Design review of the part built by this model. Coordinates are the model's own, in mm. A direction names the side the tool comes from. Coordinates: 2 decimals unless noted, no trailing zeros. Loops run counter-clockwise (first coordinate to the right, second up) from the corner with the lowest first, then second, coordinate; pieces in that order, holes last. Notation, with made-up numbers: (20, 22) - (37, 22) arc R21 cw to (37, 56) - close; hole circle Ø7 at (64, 64.25). An arc over 180 degrees is marked (long way). Answer in a Markdown table with one row per item. Add a question column.
(1) The part is to be moulded in two halves that separate along Z. For faces 3 (the face through (-19.524, 2.021, -4.336)), 4 (the face through (0, 5.6, 0)), 5 (the face through (-10.8, 2.8, -5.7)), say which applies: released by +Z, released by -Z, zero draft, split by the parting line, or undercut.
(2) We need section B-B, the plane y = 2.5. Write out the cut boundary in (x, z).
(3) We need section A-A, the plane x = 0. Write out the cut boundary in (y, z), plus the area to 3 significant figures.
(4) To check wall thickness, follow L1, parallel to X at y = 1.25, z = -6; L2, parallel to Z at x = 8, y = 4; L3, parallel to Z at x = 9.5, y = 1.8. State the ranges of each line that lie inside material, in increasing order. Write a range as [from, to].
(5) We need section D-D, the plane z = -9. Write out the cut boundary in (x, y), plus the area to 3 significant figures.
(6) Clearance check with flat-ended pins moving along their axes: pin 1 (3.5 mm diameter, centred on x = 0, z = 10, fed in from -Y); pin 2 (2 mm diameter, centred on x = -5.5, y = 2.5, fed in from -Z); pin 3 (3 mm diameter, centred on y = 2, z = -10.5, fed in from +X); pin 4 (1.5 mm diameter, centred on x = 3, y = 4.5, fed in from +Z). State where each tip first meets the part, or that it passes through.
(7) For faces 1 (the face through (-15.62, 4.84, -3.47)), 2 (the face through (0, 0, 0)), list the 3-axis set-ups (+Z, -Z, +X, -X, +Y, -Y) from which the entire face can be reached by the end or side of a thin tool; tool diameter is ignored.
(8) We need section C-C, the plane z = 0. Write out the cut boundary in (x, y).
from build123d import *

# Parameters (mm, degrees)
SKIZZE1_R                       = 20
AUFSATZ_LINEAR_AUSTRAGEN1_DEPTH = 5.6
SCHNITT_LINEAR_START            = -1.5
SKIZZE2_R                       = 20
SKIZZE2_R_2                     = 16
SCHNITT_LINEAR_AUSTRAGEN1_DEPTH = 1.5
DURCHGANGSLOCH_F_R_M41_D        = 4.5


with BuildPart() as part:
    # Skizze1 → Aufsatz-Linear austragen1 (new body)
    with BuildSketch(Plane(origin=(0, 0, 0), x_dir=(1, 0, 0), z_dir=(0, 1, 0))):
        with Locations(Location((0, 0, 0), (0, 0, 270))):
            Circle(SKIZZE1_R)
    extrude(amount=AUFSATZ_LINEAR_AUSTRAGEN1_DEPTH)

    # Skizze2 → Schnitt-Linear austragen1 (cut)
    with BuildSketch(Plane(origin=(0, 5.6, 0), x_dir=(1, 0, 0), z_dir=(0, 1, 0)).offset(SCHNITT_LINEAR_START)):
        with Locations(Location((0, 0, 0), (0, 0, 270))):
            Circle(SKIZZE2_R)
        with Locations(Location((0, 0, 0), (0, 0, 270))):
            Circle(SKIZZE2_R_2, mode=Mode.SUBTRACT)
    extrude(amount=SCHNITT_LINEAR_AUSTRAGEN1_DEPTH, mode=Mode.SUBTRACT)

    # Durchgangsloch für M41 (through all)
    with Locations(Plane(origin=(0, 5.6, 0), x_dir=(1, 0, 0), z_dir=(0, 1, 0))):
        with Locations((0, 10), (8.660254038, 5), (8.660254038, -5), (0, -10), (-8.660254038, -5), (-8.660254038, 5)):
            Hole(DURCHGANGSLOCH_F_R_M41_D / 2)


solid = part.part
Responses:
| question | item | result |
|---|---|---|
| 1 | face 3 | split by the parting line |
| 1 | face 4 | zero draft |
| 1 | face 5 | undercut |
| 2 | outline | circle Ø40 at (0, 0); hole circle Ø4.5 at (-8.66, -5); hole circle Ø4.5 at (-8.66, 5); hole circle Ø4.5 at (0, -10); hole circle Ø4.5 at (0, 10); hole circle Ø4.5 at (8.66, -5); hole circle Ø4.5 at (8.66, 5) |
| 3 | outline | (0, -20) - (4.1, -20) - (4.1, -16) - (5.6, -16) - (5.6, -12.25) - (0, -12.25) - close; (0, -7.75) - (5.6, -7.75) - (5.6, 7.75) - (0, 7.75) - close; (0, 12.25) - (5.6, 12.25) - (5.6, 16) - (4.1, 16) - (4.1, 20) - (0, 20) - close |
| 3 | area | 162 mm2 |
| 4 | L1 | x = [-19.08, -10.68], [-6.64, 6.64], [10.68, 19.08] |
| 4 | L2 | z = [-18.33, -7.15], [-2.85, 2.85], [7.15, 18.33] |
| 4 | L3 | z = [-17.6, -7.09], [-2.91, 2.91], [7.09, 17.6] |
| 5 | outline | (-17.86, 0) - (-2.02, 0) - (-2.02, 5.6) - (-13.23, 5.6) - (-13.23, 4.1) - (-17.86, 4.1) - close; (2.02, 0) - (17.86, 0) - (17.86, 4.1) - (13.23, 4.1) - (13.23, 5.6) - (2.02, 5.6) - close |
| 5 | area | 164 mm2 |
| 6 | pin 1 | passes through |
| 6 | pin 2 | stops at z = -19.49 |
| 6 | pin 3 | stops at x = 17.86 |
| 6 | pin 4 | stops at z = 19.86 |
| 7 | face 1 | +Y |
| 7 | face 2 | +Z, -Z, +X, -X, -Y |
| 8 | outline | (-20, 0) - (20, 0) - (20, 4.1) - (16, 4.1) - (16, 5.6) - (-16, 5.6) - (-16, 4.1) - (-20, 4.1) - close |
